Build history of the part. All positions in model axes, mm. A direction names the side the tool comes from. Give positions to 0.01 mm unless a question says otherwise; leave off trailing zeros. Order: outer loops, then holes, each group sorted by start corner. A loop starts at its lowest first (then second) coordinate and runs counter-clockwise, first axis right, second up. Notation, with made-up numbers: M 39.5,75 L 83.5,75 A9 cw 83.5,83 Z; hole C 71.5,12 d8. An arc over 180 degrees is marked long. Use CSV: the item, a comma, the result in double quotes. Start each with the question number.
Item 1: Band-saw the part on C-C on x = 27. Write the cut outline in (y, z) (3 decimals).
Item 2: Two-plate mould, pull along X, no slides. Class faces 1 (the flat face through (51, 60, 2)), 2 (the flat face through (7, 0, 2)), 3 (the flat face through (45, -1, 2)): pulls with the +X half, pulls with the -X half, needs draft (parallel to the pull), parting line crosses it, or undercut.
Item 3: Wall check: line 1 along X through (y, z) = (79, 2.2); line 2 along X through (y, z) = (49, 0.55); line 3 along Y through (x, z) = (6.5, 2.05). Give the ranges that are in metal, low to high.
Item 4: Pin check, flat tips, straight feed: P1, Ø1.2, axis at x = 51, z = 2, coming from the +Y side; P2, Ø1.6, axis at x = 8, z = 1.5, coming from the -Y side; P3, Ø1.6, axis at y = 48, z = 2, coming from the +X side. Stop position of each tip, or through.
Item 5: Band-saw the part on A-A on x = 9. Write the cut outline in (y, z) (3 decimals).
Item 6: Which spindle directions (+Z, -Z, +X, -X, +Y, -Y) get a long thin tool onto all of the face, cutting with end or side? Do faces 4 (the flat face through (2, -2.5, 2)), 5 (the flat face through (51, 40, 2)), 6 (the flat face through (50, 87, 2)), 7 (the flat face through (5, -1, 2)), 8 (the flat face through (52.5, 53, 2)). Say none if no direction does.
Item 7: Band-saw the part on B-B on y = 37.5. Write the cut outline in (x, z) (3 decimals).
from build123d import *

# Parameters (mm, degrees)
SKETCH1_W           = 50
SKETCH1_H           = 90
BOSS_EXTRUDE2_DEPTH = 3.175
SKETCH2_W           = 3.175
SKETCH2_H           = 5
BOSS_EXTRUDE3_DEPTH = 2.5
LPATTERN1_COUNT     = 9
LPATTERN1_PITCH     = 10
SKETCH3_W           = 5
SKETCH3_H           = 3.175
BOSS_EXTRUDE4_DEPTH = 2.5
LPATTERN2_COUNT     = 5
LPATTERN2_PITCH     = 10
SKETCH4_R           = 2.5
CUT_EXTRUDE1_DEPTH  = 10


with BuildPart() as part:
    # Sketch1 → Boss-Extrude2 (new body)
    with BuildSketch(Plane.XY):
        with Locations((25, 45)):
            Rectangle(SKETCH1_W, SKETCH1_H)
    extrude(amount=BOSS_EXTRUDE2_DEPTH)

    # Sketch2 → Boss-Extrude3 (add)
    with BuildSketch(Plane(origin=(50, 0, 0), x_dir=(0, 0, -1), z_dir=(1, 0, 0))):
        with Locations((-1.5875, 2.5)):
            Rectangle(SKETCH2_W, SKETCH2_H)
    boss_extrude3 = extrude(amount=BOSS_EXTRUDE3_DEPTH)

    # LPattern1: Boss-Extrude3 ×9
    with Locations(*[(0, i * LPATTERN1_PITCH, 0) for i in range(1, LPATTERN1_COUNT)]):
        add(boss_extrude3)

    # Sketch3 → Boss-Extrude4 (add)
    with BuildSketch(Plane.XZ):
        with Locations((2.5, 1.5875)):
            Rectangle(SKETCH3_W, SKETCH3_H)
    boss_extrude4 = extrude(amount=BOSS_EXTRUDE4_DEPTH)

    # LPattern2: Boss-Extrude4 ×5
    with Locations(*[(i * LPATTERN2_PITCH, 0, 0) for i in range(1, LPATTERN2_COUNT)]):
        add(boss_extrude4)

    # Sketch4 → Cut-Extrude1 (cut)
    with BuildSketch(Plane.XY.offset(3.175)):
        with Locations((10, 80)):
            Circle(SKETCH4_R)
    extrude(amount=-CUT_EXTRUDE1_DEPTH, mode=Mode.SUBTRACT)


solid = part.part
Model answer:
1,outline,"M 0,0 L 90,0 L 90,3.175 L 0,3.175 Z"
2,face 1,"needs draft"
2,face 2,"undercut"
2,face 3,"pulls with the +X half"
3,line 1,"x = 0 to 7.71, 12.29 to 50"
3,line 2,"x = 0 to 50"
3,line 3,"y = 0 to 90"
4,P1,"stops at y = 85"
4,P2,"stops at y = 0"
4,P3,"stops at x = 50"
5,outline,"M 0,0 L 77.709,0 L 77.709,3.175 L 0,3.175 Z; M 82.291,0 L 90,0 L 90,3.175 L 82.291,3.175 Z"
6,face 4,"+Z, -Z, +X, -X, -Y"
6,face 5,"+Z, -Z, +X"
6,face 6,"+Z, -Z, +X, +Y"
6,face 7,"+Z, -Z, -Y"
6,face 8,"+Z, -Z, +X, +Y, -Y"
7,outline,"M 0,0 L 50,0 L 50,3.175 L 0,3.175 Z"
